Could you check a few things on this model? Use its own coordinates, in mm. Face numbers are marked on the shaded views. A direction names the side the tool comes from. Round coordinates to 2 decimals unless told otherwise and drop trailing zeros. Write each loop counter-clockwise with the first axis right and the second up, starting at its lowest first coordinate (ties: lowest second). Pieces come first, ordered by that corner, then holes. Notation, with made-up numbers: (-27, 65) -> (11, 65) arc R16 cw to (11, 69) -> close; hole circle Ø11 at (80, 31.25). An arc over 180 degrees is marked (long way). Answer as CSV lines item,"result". Start each with the question number.
Q1. Imagine slicing it at B-B on z = -15. Please give me the cut outline in (x, y), and give its area (3 significant figures).
Q2. For the marked faces 1, 2 and 3, which set-ups out of +Z, -Z, +X, -X, +Y, -Y let a thin tool reach every point of the face, with its end or its side?
Q3. If I drill on line 1 (X direction, y = 8, z = 3); line 2 (Z direction, x = 39, y = 45); line 3 (Y direction, x = 47.5, z = 30.5), over which ranges is the centre line in solid material (lowest first)? Write a range as [from, to].
Q4. Imagine slicing it at A-A on x = 8. Please give me the cut outline in (y, z).
Q5. Will these pins go through, and if not, where does the flat tip stop? pin 1 Ø6 at (x, z) = (24, 3.5) entering from +Y; pin 2 Ø3 at (x, y) = (30, -2) entering from -Z; pin 3 Ø4.5 at (y, z) = (-1.5, -73.5) entering from +X.
Q6. Imagine slicing it at C-C on y = 102.5. Please give me the cut outline in (x, z).
Q7. Imagine slicing it at D-D on z = 4. Please give me the cut outline in (x, y), and give its area (3 significant figures).
from build123d import *

# Parameters (mm, degrees)
F0_W     = 90
F0_H     = 50
F0_H_2   = 30
F0_R     = 1.55
F0_W_2   = 19
F0_H_3   = 3
F1_DEPTH = 4
F3_DEPTH = 4
F4_W     = 0.5
F4_H     = 20
F5_DEPTH = 0.5


with BuildPart() as f1:
    # F0 (on Front) → F1 (new body)
    with BuildSketch(Plane.XZ):
        Polygon((50.859297, 66.157015), (-49.140703, 66.157015), (-49.140703, -63.842985), (-9.140703, -63.842985), (-9.140703, -83.842985), (10.859297, -83.842985), (10.859297, -63.842985), (50.859297, -63.842985), align=None)
        with Locations((0.859297, -28.842985)):
            Rectangle(F0_W, F0_H, mode=Mode.SUBTRACT)
        with Locations((0.859297, 21.157015)):
            Rectangle(F0_W, F0_H_2, mode=Mode.SUBTRACT)
        with Locations((-26.640703, 41.357015)):
            Circle(F0_R, mode=Mode.SUBTRACT)
        with Locations((-18.640703, 41.357015)):
            Circle(F0_R, mode=Mode.SUBTRACT)
        with Locations((0.859297, 57.657015)):
            Rectangle(F0_W_2, F0_H_3, mode=Mode.SUBTRACT)
        with Locations((20.359297, 56.357015)):
            Circle(F0_R, mode=Mode.SUBTRACT)
        with Locations((28.359297, 56.357015)):
            Circle(F0_R, mode=Mode.SUBTRACT)
    extrude(amount=F1_DEPTH)

    # F2 (on face) → F3 (join)
    with BuildSketch(Plane.XY.offset(6.157015)):
        with BuildLine():
            Line((-49.140703, 105), (-49.140703, 0))
            Line((-49.140703, 0), (-29.140703, 0))
            Line((-29.140703, 0), (-29.140703, 105))
            ThreePointArc((-29.140703, 105), (-30.605169, 108.535534), (-34.140703, 110))
            Line((-34.140703, 110), (-44.140703, 110))
            ThreePointArc((-44.140703, 110), (-47.676237, 108.535534), (-49.140703, 105))
        make_face()
        Polygon((-46.854805, 62), (-43.390703, 64), (-39.926602, 62), (-39.926602, 58), (-43.390703, 56), (-46.854805, 58), align=None, mode=Mode.SUBTRACT)
        with BuildLine():
            Line((30.859297, 105), (30.859297, 0))
            Line((30.859297, 0), (50.859297, 0))
            Line((50.859297, 0), (50.859297, 105))
            ThreePointArc((50.859297, 105), (49.394831, 108.535534), (45.859297, 110))
            Line((45.859297, 110), (35.859297, 110))
            ThreePointArc((35.859297, 110), (32.323763, 108.535534), (30.859297, 105))
        make_face()
        Polygon((45.109297, 64), (48.573398, 62), (48.573398, 58), (45.109297, 56), (41.645195, 58), (41.645195, 62), align=None, mode=Mode.SUBTRACT)
    extrude(amount=-F3_DEPTH)

    # F4 (on face) → F5 (cut)
    with BuildSketch(Plane(origin=(0, 0, 0), x_dir=(-1, 0, 0), z_dir=(0, 1, 0))):
        with Locations((-0.859297, -73.842985)):
            Rectangle(F4_W, F4_H)
    extrude(amount=-F5_DEPTH, mode=Mode.SUBTRACT)


solid = f1.part
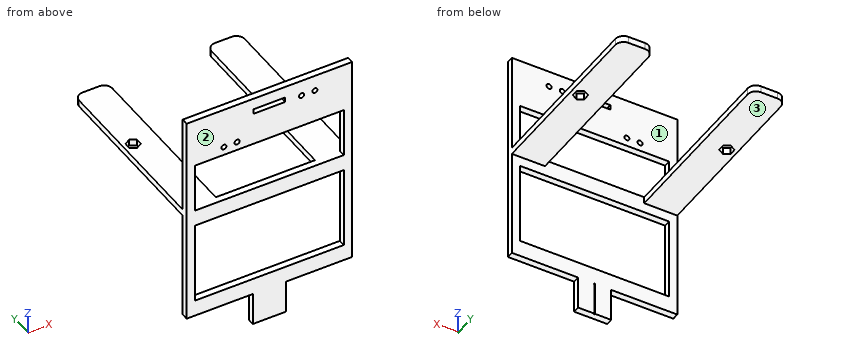
Checks:
1,outline,"(-49.14, -4) -> (-44.14, -4) -> (-44.14, 0) -> (-49.14, 0) -> close; (45.86, -4) -> (50.86, -4) -> (50.86, 0) -> (45.86, 0) -> close"
1,area,"40.0 mm^2"
2,face 1,"+Z, +X, -X, +Y"
2,face 2,"+Z, -Z, +X, -X, -Y"
2,face 3,"-Z, +X, -X, +Y"
3,line 1,"[-49.14, -29.14], [30.86, 50.86]"
3,line 2,"[2.16, 6.16]"
3,line 3,"[-4, 0]"
4,outline,"(-4, -83.84) -> (0, -83.84) -> (0, -53.84) -> (-4, -53.84) -> close; (-4, -3.84) -> (0, -3.84) -> (0, 6.16) -> (-4, 6.16) -> close; (-4, 36.16) -> (0, 36.16) -> (0, 56.16) -> (-4, 56.16) -> close; (-4, 59.16) -> (0, 59.16) -> (0, 66.16) -> (-4, 66.16) -> close"
5,pin 1,"y = 0"
5,pin 2,"z = -63.84"
5,pin 3,"x = 10.86"
6,outline,"(-49.14, 2.16) -> (-29.14, 2.16) -> (-29.14, 6.16) -> (-49.14, 6.16) -> close; (30.86, 2.16) -> (50.86, 2.16) -> (50.86, 6.16) -> (30.86, 6.16) -> close"
7,outline,"(-49.14, -4) -> (50.86, -4) -> (50.86, 105) arc R5 ccw to (45.86, 110) -> (35.86, 110) arc R5 ccw to (30.86, 105) -> (30.86, 0) -> (-29.14, 0) -> (-29.14, 105) arc R5 ccw to (-34.14, 110) -> (-44.14, 110) arc R5 ccw to (-49.14, 105) -> close; hole (-46.85, 58) -> (-43.39, 56) -> (-39.93, 58) -> (-39.93, 62) -> (-43.39, 64) -> (-46.85, 62) -> close; hole (41.65, 58) -> (45.11, 56) -> (48.57, 58) -> (48.57, 62) -> (45.11, 64) -> (41.65, 62) -> close"
7,area,"4,700 mm^2"
